from build123d import *

# Parameters (mm, degrees)
BASE_EXTRUDE_START                = -81.5
BASE_EXTRUDE_DEPTH                = 81.5
SKETCH2_R                         = 10
CUT_EXTRUDE1_DEPTH                = 80.2
SKETCH4_R                         = 10
BOSS_EXTRUDE1_DEPTH               = 10
CUT_EXTRUDE3_REACH                = 88.633
SKETCH19_R                        = 5
F_1_4_20_TAPPED_HOLE1_D           = 5.1054
F_1_4_20_TAPPED_HOLE1_DEPTH       = 18.288
F_1_4_20_TAPPED_HOLE1_CBORE_D     = 6.35
F_1_4_20_TAPPED_HOLE1_CBORE_DEPTH = 11.938
F_1_4_20_TAPPED_HOLE1_TIP         = 1.533816902
F_10_32_TAPPED_HOLE2_D            = 4.0386
F_10_32_TAPPED_HOLE2_DEPTH        = 13.8684
F_10_32_TAPPED_HOLE2_CBORE_D      = 4.826
F_10_32_TAPPED_HOLE2_CBORE_DEPTH  = 9.906
F_10_32_TAPPED_HOLE2_TIP          = 1.213317848
HOLE1_D                           = 5
HOLE1_DEPTH                       = 5
CUT_EXTRUDE4_DEPTH                = 5
F_10_32_TAPPED_HOLE1_D            = 4.0386
F_10_32_TAPPED_HOLE1_DEPTH        = 13.6144
F_10_32_TAPPED_HOLE1_CBORE_D      = 4.826
F_10_32_TAPPED_HOLE1_CBORE_DEPTH  = 9.652
F_10_32_TAPPED_HOLE1_TIP          = 1.213317848
SKETCH30_W                        = 40
SKETCH30_H                        = 47
BOSS_EXTRUDE2_DEPTH               = 12
BOSS_EXTRUDE3_DEPTH               = 3
SKETCH35_R                        = 3.5
BOSS_EXTRUDE5_DEPTH               = 5
CHAMFER2_SIZE                     = 0.5
BOSS_EXTRUDE6_DEPTH               = 12
BOSS_EXTRUDE7_DEPTH               = 3
CUT_EXTRUDE7_REACH                = 121.044
SKETCH38_R                        = 7
CUT_EXTRUDE8_REACH                = 179.193
SKETCH46_R                        = 7
CHAMFER3_SIZE                     = 2


with BuildPart() as part:
    # Sketch1 → Base-Extrude (new body)
    with BuildSketch(Plane(origin=(0, 0, 48.65), x_dir=(-1, 0, 0), z_dir=(0, 0, 1)).offset(BASE_EXTRUDE_START)):
        with BuildLine():
            Line((31.365, 12.6873), (32, 12.0523))
            Line((32, 12.0523), (32, -12.0523))
            Line((32, -12.0523), (31.365, -12.6873))
            Line((31.365, -12.6873), (9.271, -12.6873))
            Line((9.271, -12.6873), (8.636, -12.0523))
            Line((8.636, -12.0523), (-8.636, -12.0523))
            Line((-8.636, -12.0523), (-9.271, -12.6873))
            Line((-9.271, -12.6873), (-31.365, -12.6873))
            Line((-31.365, -12.6873), (-32, -12.0523))
            Line((-32, -12.0523), (-32, -6.7691))
            Line((-32, -6.7691), (-30.791853982, -6.7691))
            ThreePointArc((-30.791853982, -6.7691), (-27.209184534, -5.2324), (-30.791853982, -3.6957))
            Line((-30.791853982, -3.6957), (-32, -3.6957))
            Line((-32, -3.6957), (-32, 3.6957))
            Line((-32, 3.6957), (-30.791853982, 3.6957))
            ThreePointArc((-30.791853982, 3.6957), (-27.209184534, 5.2324), (-30.791853982, 6.7691))
            Line((-30.791853982, 6.7691), (-32, 6.7691))
            Line((-32, 6.7691), (-32, 12.0523))
            Line((-32, 12.0523), (-31.365, 12.6873))
            Line((-31.365, 12.6873), (-9.271, 12.6873))
            Line((-9.271, 12.6873), (-8.636, 12.0523))
            Line((-8.636, 12.0523), (8.636, 12.0523))
            Line((8.636, 12.0523), (9.271, 12.6873))
            Line((9.271, 12.6873), (31.365, 12.6873))
        make_face()
    extrude(amount=BASE_EXTRUDE_DEPTH)

    # Sketch2 → Cut-Extrude1 (cut)
    with BuildSketch(Plane(origin=(0, 0, 48.65), x_dir=(-1, 0, 0), z_dir=(0, 0, -1))):
        with Locations(Location((-16.4592, 0, 0), (0, 0, 180))):
            Circle(SKETCH2_R)
        with Locations(Location((14.9352, 0, 0), (0, 0, 180))):
            Circle(SKETCH2_R)
    extrude(amount=CUT_EXTRUDE1_DEPTH, mode=Mode.SUBTRACT)

    # Sketch4 → Boss-Extrude1 (add)
    with BuildSketch(Plane.XY.offset(46.65)):
        with Locations((16.4592, 0)):
            Circle(SKETCH4_R)
        with Locations((-14.9352, 0)):
            Circle(SKETCH4_R)
    extrude(amount=-BOSS_EXTRUDE1_DEPTH)

    # Sketch19 → Cut-Extrude3 (cut, up to next)
    with BuildSketch(Plane.XY.offset(46.65), mode=Mode.PRIVATE) as cut_extrude3_sk1:
        with Locations((16.4592, 0)):
            Circle(SKETCH19_R)
    cut_extrude3_tool1 = extrude(cut_extrude3_sk1.sketch, amount=-CUT_EXTRUDE3_REACH, mode=Mode.PRIVATE) & part.part
    # Sketch19 → Cut-Extrude3 (cut, up to next)
    with BuildSketch(Plane.XY.offset(46.65), mode=Mode.PRIVATE) as cut_extrude3_sk2:
        with Locations((-14.9352, 0)):
            Circle(SKETCH19_R)
    cut_extrude3_tool2 = extrude(cut_extrude3_sk2.sketch, amount=-CUT_EXTRUDE3_REACH, mode=Mode.PRIVATE) & part.part
    add(cut_extrude3_tool1.solids().sort_by_distance((16.4592, 0, 46.65))[0], mode=Mode.SUBTRACT)
    add(cut_extrude3_tool2.solids().sort_by_distance((-14.9352, 0, 46.65))[0], mode=Mode.SUBTRACT)

    # 1/4-20 Tapped Hole1
    with Locations(Plane.XZ.offset(12.0523)):
        with Locations((0, 23.15), (0, -6.85)):
            CounterBoreHole(F_1_4_20_TAPPED_HOLE1_D / 2, F_1_4_20_TAPPED_HOLE1_CBORE_D / 2, F_1_4_20_TAPPED_HOLE1_CBORE_DEPTH, depth=F_1_4_20_TAPPED_HOLE1_DEPTH)
            with Locations((0, 0, -(F_1_4_20_TAPPED_HOLE1_DEPTH + F_1_4_20_TAPPED_HOLE1_TIP / 2))):  # 118° drill point
                Cone(0, F_1_4_20_TAPPED_HOLE1_D / 2, F_1_4_20_TAPPED_HOLE1_TIP, mode=Mode.SUBTRACT)

    # #10-32 Tapped Hole2
    with Locations(Plane(origin=(0, 0, -32.85), x_dir=(-1, 0, 0), z_dir=(0, 0, -1))):
        with Locations((28, -7.5873), (28, 7.8127), (-4.5, -7.5873), (-4.5, 7.8127)):
            CounterBoreHole(F_10_32_TAPPED_HOLE2_D / 2, F_10_32_TAPPED_HOLE2_CBORE_D / 2, F_10_32_TAPPED_HOLE2_CBORE_DEPTH, depth=F_10_32_TAPPED_HOLE2_DEPTH)
            with Locations((0, 0, -(F_10_32_TAPPED_HOLE2_DEPTH + F_10_32_TAPPED_HOLE2_TIP / 2))):  # 118° drill point
                Cone(0, F_10_32_TAPPED_HOLE2_D / 2, F_10_32_TAPPED_HOLE2_TIP, mode=Mode.SUBTRACT)

    # Hole1
    with Locations(Plane.XZ.offset(12.6873)):
        with Locations((-27.5, 36.15)):
            Hole(HOLE1_D / 2, depth=HOLE1_DEPTH)

    # Sketch27 → Cut-Extrude4 (cut)
    with BuildSketch(Plane.XZ.offset(12.6873)):
        with BuildLine():
            Line((-30, -13.35), (-30, -14.35))
            ThreePointArc((-30, -14.35), (-27.5, -16.85), (-25, -14.35))
            Line((-25, -14.35), (-25, -13.35))
            ThreePointArc((-25, -13.35), (-27.5, -10.85), (-30, -13.35))
        make_face()
    extrude(amount=-CUT_EXTRUDE4_DEPTH, mode=Mode.SUBTRACT)

    # #10-32 Tapped Hole1
    with Locations(Plane.ZY.offset(32)):
        with Locations((27.85, -0.1873), (-24.85, -0.1873)):
            CounterBoreHole(F_10_32_TAPPED_HOLE1_D / 2, F_10_32_TAPPED_HOLE1_CBORE_D / 2, F_10_32_TAPPED_HOLE1_CBORE_DEPTH, depth=F_10_32_TAPPED_HOLE1_DEPTH)
            with Locations((0, 0, -(F_10_32_TAPPED_HOLE1_DEPTH + F_10_32_TAPPED_HOLE1_TIP / 2))):  # 118° drill point
                Cone(0, F_10_32_TAPPED_HOLE1_D / 2, F_10_32_TAPPED_HOLE1_TIP, mode=Mode.SUBTRACT)

    # Sketch30 → Boss-Extrude2 (add)
    with BuildSketch(Plane(origin=(0, 0, -32.85), x_dir=(-1, 0, 0), z_dir=(0, 0, -1))):
        with Locations((11, 11.9477)):
            Rectangle(SKETCH30_W, SKETCH30_H)
    extrude(amount=BOSS_EXTRUDE2_DEPTH)

    # Sketch31 → Boss-Extrude3 (add)
    with BuildSketch(Plane(origin=(0, 0, -44.85), x_dir=(-1, 0, 0), z_dir=(0, 0, -1))):
        Polygon((25.237604307, 25.4477), (20.618802154, 33.4477), (11.381197846, 33.4477), (6.762395693, 25.4477), (11.381197846, 17.4477), (20.618802154, 17.4477), align=None)
    extrude(amount=BOSS_EXTRUDE3_DEPTH)

    # Sketch35 → Boss-Extrude5 (add)
    with BuildSketch(Plane(origin=(0, 0, -44.85), x_dir=(-1, 0, 0), z_dir=(0, 0, -1))):
        with Locations(Location((28, 7.8127, 0), (0, 0, 328.997280866))):
            Circle(SKETCH35_R)
        with Locations((-4.5, 7.8127)):
            Circle(SKETCH35_R)
        with Locations((-4.5, -7.5873)):
            Circle(SKETCH35_R)
        with Locations(Location((28, -7.5873, 0), (0, 0, 328.997280866))):
            Circle(SKETCH35_R)
    extrude(amount=BOSS_EXTRUDE5_DEPTH)

    # Chamfer2
    chamfer2_edges = [part.edges().sort_by_distance(p)[0] for p in [
        (-25, 9.615475638, -49.85),
        (8, 7.8127, -49.85),
        (8, -7.5873, -49.85),
        (-25, -5.784524362, -49.85),
    ]]
    chamfer(chamfer2_edges, length=CHAMFER2_SIZE)

    # Sketch36 → Boss-Extrude6 (add)
    with BuildSketch(Plane.XY.offset(34.65)):
        Polygon((-32.5, 36.8127), (-32.5, 10.6873), (-32, 10.6873), (-32, -10.6873), (-54, -10.6873), (-54, 36.8127), align=None)
    extrude(amount=BOSS_EXTRUDE6_DEPTH)

    # Sketch37 → Boss-Extrude7 (add)
    with BuildSketch(Plane.XY.offset(46.65)):
        Polygon((-39.381197846, 34.8127), (-48.618802154, 34.8127), (-53.237604307, 26.8127), (-48.618802154, 18.8127), (-39.381197846, 18.8127), (-34.762395693, 26.8127), align=None)
    extrude(amount=BOSS_EXTRUDE7_DEPTH)

    # Sketch38 → Cut-Extrude7 (cut, up to next)
    with BuildSketch(Plane.XY.offset(49.65), mode=Mode.PRIVATE) as cut_extrude7_sk1:
        with Locations((-44, 26.8127)):
            Circle(SKETCH38_R)
    cut_extrude7_tool1 = extrude(cut_extrude7_sk1.sketch, amount=-CUT_EXTRUDE7_REACH, mode=Mode.PRIVATE) & part.part
    add(cut_extrude7_tool1.solids().sort_by_distance((-44, 26.8127, 49.65))[0], mode=Mode.SUBTRACT)

    # Sketch44 → Boss-Revolve1 (revolve)
    with BuildSketch(Plane(origin=(0, 26.8127, 0), x_dir=(-1, 0, 0), z_dir=(0, 1, 0)), mode=Mode.PRIVATE) as boss_revolve1_sk:
        Polygon((44, 116.85), (51, 116.85), (51, 36.65), (49, 34.65), (44, 34.65), align=None)
    revolve(boss_revolve1_sk.sketch.rotate(Axis((-44, 26.8127, 49.65), (0, 0, -1)), 180), axis=Axis((-44, 26.8127, 49.65), (0, 0, -1)))

    # Sketch46 → Cut-Extrude8 (cut, up to next)
    with BuildSketch(Plane(origin=(0, 0, -47.85), x_dir=(-1, 0, 0), z_dir=(0, 0, -1)), mode=Mode.PRIVATE) as cut_extrude8_sk1:
        with Locations((16, 25.4477)):
            Circle(SKETCH46_R)
    cut_extrude8_tool1 = extrude(cut_extrude8_sk1.sketch, amount=-CUT_EXTRUDE8_REACH, mode=Mode.PRIVATE) & part.part
    add(cut_extrude8_tool1.solids().sort_by_distance((-16, 25.4477, -47.85))[0], mode=Mode.SUBTRACT)

    # Sketch47 → Boss-Revolve2 (revolve)
    with BuildSketch(Plane(origin=(0, 25.4477, 0), x_dir=(-1, 0, 0), z_dir=(0, 1, 0))):
        Polygon((21, -32.85), (16, -32.85), (16, -115.05), (23, -115.05), (23, -34.85), align=None)
    revolve(axis=Axis((-16, 25.4477, -32.85), (0, 0, -1)))

    # Chamfer3
    chamfer3_edges = [part.edges().sort_by_distance(p)[0] for p in [
        (-51, 26.8127, 116.85),
        (-9, 25.4477, -115.05),
    ]]
    chamfer(chamfer3_edges, length=CHAMFER3_SIZE)


solid = part.part
Read the model definition and answer for the solid it produces. Units are mm, in the model's axes. A direction names the side the tool comes from. Give positions to 0.01 mm unless a question says otherwise; leave off trailing zeros. Loops run counter-clockwise (first coordinate to the right, second up) from the corner with the lowest first, then second, coordinate; pieces in that order, holes last. Notation, with made-up numbers: M 3,-1 L 43,-1 A6 ccw 43,9 Z; hole C 28,38 d5. An arc over 180 degrees is marked long. Write each question's results on one line, items separated by ' | '.
1. A tool of negligible diameter and unlimited length cuts with its end or side. For faces 5 (the face through (-50.896, 30.869, 48.129)), 6 (the face through (-37.323, 24.71, 81.794)), 7 (the face through (-2, -0.114, -5)), 8 (the face through (8.52, 6.08, 3.03)), 9 (the face through (-43, 13, 34.65)), from which of +Z, -Z, +X, -X, +Y, -Y can it reach the whole face along a straight path? Write none if from no direction.
Values:
face 5: +Z, -X, +Y | face 6: +Z | face 7: -Y | face 8: none | face 9: -Z, -X, +Y, -Y
2. Section A-A on x = -44 is taken. Give the vertices of the cut face in (y, z).
Values:
outline: M -10.69,34.65 L 19.81,34.65 L 19.81,36.65 L 21.81,34.65 L 31.81,34.65 L 33.81,36.65 L 33.81,34.65 L 36.81,34.65 L 36.81,46.65 L 34.81,46.65 L 34.81,49.65 L 33.81,49.65 L 33.81,114.85 L 31.81,116.85 L 21.81,116.85 L 19.81,114.85 L 19.81,49.65 L 18.81,49.65 L 18.81,46.65 L -10.69,46.65 Z
3. Section B-B on z = 57 is taken. Give the vertices of the cut face in (x, y).
Values:
outline: C -44,26.81 d14
4. Given pin 1 (1.8 mm diameter, centred on x = 5, y = -7.5, fed in from -Z); pin 2 (1.5 mm diameter, centred on x = -6, z = -44.5, fed in from -Y); pin 3 (4.5 mm diameter, centred on x = -28, y = -7.59, fed in from +Z); pin 4 (8 mm diameter, centred on y = 14.5, z = 87.5, fed in from -X), each flat-ended and moving along its own axis, determine where each tip first touches the part or whether it passes through.
Values:
pin 1: stops at z = -49.85 | pin 2: stops at y = -11.55 | pin 3: stops at z = 48.65 | pin 4: passes through
5. Straight lines are drawn through the part: line 1 (Z direction, x = -27.5, y = -10.3); line 2 (Y direction, x = -28, z = -21.05); line 3 (X direction, y = 2.5, z = 7). For each, find the intervals that lie inside material, in ascending order. Write a range as [from, to].
Values:
line 1: z = [-49.85, -16.85], [-10.85, 33.65], [38.65, 48.65] | line 2: y = [-12.69, -9.61], [-5.57, 5.79], [9.83, 12.69] | line 3: x = [-32, -24.62], [-5.25, 6.78], [26.14, 32]
6. The mould has two halves that part along Y. Classify faces 1 (the face through (-28, -8, -49.85)), 2 (the face through (-0.058, 7.503, 23.59)), 3 (the face through (-28.34, 0.54, 30.15)), 4 (the face through (19, 5, 36.65)): pulls with the +Y half, pulls with the -Y half, needs draft (parallel to the pull), parting line crosses it, or undercut.
Values:
face 1: needs draft | face 2: pulls with the -Y half | face 3: undercut | face 4: undercut
